The model under review builds one solid part; all positions refer to its coordinate system, in mm. A direction names the side the tool comes from. Round coordinates to 2 decimals unless told otherwise and drop trailing zeros. Loops run counter-clockwise (first coordinate to the right, second up) from the corner with the lowest first, then second, coordinate; pieces in that order, holes last. Notation, with made-up numbers: M 57.25,-31.5 L 70.25,-31.5 A25 cw 70.25,7.5 Z; hole C 48,-9 d6. An arc over 180 degrees is marked long. Return JSON: item names as keys, results as strings. Group by question number.
Q1. Draft analysis for pull direction Y (two halves, no side actions). For faces 1 (the face through (8.909, -0.885, 38.809)), 2 (the face through (-0.9, 8.91, 32.47)), 3 (the face through (7.9, -2.49, 11.74)), state which applies: pulls with the +Y half, pulls with the -Y half, needs draft (parallel to the pull), parting line crosses it, or undercut.
Q2. Consider section C-C (z = 13). State the section outline as (x, y) points.
Q3. Clearance check with flat-ended pins moving along their axes: pin 1 Ø4 at (x, y) = (5.5, 5) entering from +Z; pin 2 Ø2 at (y, z) = (-8, 47.5) entering from +X; pin 3 Ø1 at (x, y) = (0, -14) entering from -Z. State where each tip first meets the part, or that it passes through.
Q4. To check wall thickness, follow line 1 along Y through (x, z) = (5.25, 60.5); line 2 along Y through (x, z) = (0, 20); line 3 along Y through (x, z) = (-5.5, 10). State the ranges of each line that lie inside material, in increasing order.
Q5. For faces 4 (the face through (8, 41, 30.172)), 5 (the face through (6, 7, 49.212)), 6 (the face through (0, -8.282, 27)), 7 (the face through (4.3, -4.9, 61.912)), list the 3-axis set-ups (+Z, -Z, +X, -X, +Y, -Y) from which the entire face can be reached by the end or side of a thin tool; tool diameter is ignored.
Q6. Consider section B-B (y = 55). State the section outline as (x, z) points, and give its area (3 significant figures).
Autodesk Inventor part; units mm, degrees
ref_plane "YZ Plane" through (0, 0, 0) normal (1, 0, 0) x (0, 1, 0)
ref_plane "XZ Plane" through (0, 0, 0) normal (0, 1, 0) x (-1, 0, 0)
ref_plane "XY Plane" through (0, 0, 0) normal (0, 0, 1) x (1, 0, 0)
sketch "Sketch1" plane through (0, 0, 0) normal (0, 0, 1) x (1, 0, 0)
  circle A0 centre (0, 0) radius 6.35
  circle A1 centre (0, 0) radius 8.2824
  dimension "d0" = 12.7
extrude "Extrusion1" add sketch "Sketch1" along normal blind 23.8125
sketch "Sketch2" plane through (0, 0, 23.8125) normal (0, 0, 1) x (1, 0, 0)
  circle A0 centre (0, 0) radius 6.35
  circle A1 centre (0, 0) radius 8.2824
  line L0 (8.2824, 8.2824) -> (-8.2824, 8.2824)
  line L1 (-8.2824, -8.2824) -> (8.2824, -8.2824)
  line L2 (8.2824, -8.2824) -> (8.2824, 8.2824)
  line L3 (-8.2824, 8.2824) -> (-8.2824, -8.2824)
  circle A2 centre (0, 0) radius 6.35
extrude "Extrusion2" add sketch "Sketch2" along normal blind 25.4
sketch "Sketch3" plane through (0, 0, 49.2125) normal (0, 0, 1) x (1, 0, 0)
  circle A0 centre (0, 0) radius 6.35
  circle A1 centre (0, 0) radius 6.35
  circle A2 centre (0, 0) radius 8.2824
extrude "Extrusion3" add sketch "Sketch3" along normal blind 12.7
sketch "Sketch4" plane through (8.2824, -8.2824, 23.8125) normal (1, 0, 0) x (0, 0, -1)
  line L0 (-15.8821, 8.2824) -> (-14.086, 10.0784)
  line L1 (-15.8821, 8.2824) -> (-13.3421, 8.2824) construction
  line L2 (-14.086, 10.0784) -> (-14.086, 9.1804)
  line L3 (-15.8821, 8.2824) -> (-14.086, 6.4863)
  line L4 (-14.086, 6.4863) -> (-14.086, 7.3843)
  line L5 (-14.086, 7.3843) -> (-9.4174, 7.3843)
  line L6 (-9.4174, 7.3843) -> (-9.4174, 9.1804)
  line L7 (-9.4174, 9.1804) -> (-14.086, 9.1804)
  point P0 (23.8125, 8.2824)
  dimension "d7" = 2.54
  dimension "d8" = 45
extrude "Extrusion4" add sketch "Sketch4" along normal blind 1.27
sketch "Sketch5" plane through (0, 8.2824, 23.8125) normal (0, 1, 0) x (1, 0, 0)
  circle A0 centre (0, -12.7) radius 4.1412
  point P0 (0, 23.8125)
extrude "Extrusion5" add sketch "Sketch5" along normal blind 1.27
sketch "Sketch6" plane through (0, 9.5524, 36.5125) normal (0, 1, 0) x (1, 0, 0)
  circle A0 centre (0, 0) radius 4.1412
  circle A1 centre (0, 0) radius 7.62
  point P0 (0, 36.5125)
  dimension "d13" = 15.24
extrude "Extrusion6" add sketch "Sketch6" along normal blind 50.8 contours A0 | A1
sketch "Sketch7" plane through (0, 8.2824, 23.8125) normal (0, 1, 0) x (1, 0, 0)
  line L0 (8.2824, 0) -> (8.2824, -25.4)
  line L1 (8.2824, -19.0619) -> (8.2824, -6.3591)
  line L2 (8.2824, -6.3591) -> (7.0124, -6.3591)
  line L3 (7.0124, -6.3591) -> (7.0124, -19.0619)
  line L4 (7.0124, -19.0619) -> (8.2824, -19.0619)
  point P0 (0, 23.8125)
  dimension "d16" = 1.27
extrude "Extrusion7" add sketch "Sketch7" along normal blind 53.34
sketch "Sketch8" plane through (7.0124, 8.2824, 30.1716) normal (-1, 0, 0) x (0, 0, 1)
  line L0 (12.7028, 0) -> (12.7028, 53.34)
  line L1 (0, 53.34) -> (12.7028, 53.34)
  line L2 (12.7028, 53.34) -> (12.7028, 52.07)
  line L3 (12.7028, 52.07) -> (0, 52.07)
  line L4 (0, 52.07) -> (0, 53.34)
  point P0 (-30.1716, -8.2824)
  dimension "d19" = 1.27
extrude "Extrusion8" add sketch "Sketch8" along normal blind 12.7
sketch "Sketch9" plane through (-8.2824, -8.2824, 23.8125) normal (0, -1, 0) x (1, 0, 0)
  line L0 (0, 0) -> (0, 25.4)
  line L1 (16.5647, 0) -> (16.5647, 25.4)
  circle A0 centre (8.2824, 12.7) radius 8.2824
  line L2 (0, 21.8506) -> (16.5647, 21.8506)
  point P0 (8.2824, -23.8125)
revolve "Revolution1" add sketch "Sketch9" angle 45 about axis through (-8.2824, -8.2824, 45.6631) along (-1, 0, 0) contours A0
sketch "Sketch10" plane through (0, -14.7528, 39.1926) normal (0, -0.7071, 0.7071) x (-1, 0, 0)
  circle A0 centre (0, 0) radius 8.2824
  circle A1 centre (0, 0) radius 8.2824
  point P0 (0, 17.2816)
extrude "Extrusion9" add sketch "Sketch10" along normal blind 25.4
thread "Thread1"
properties part number "solenoid valve"
Values:
{
 "1": {"face 1": "pulls with the -Y half", "face 2": "undercut", "face 3": "parting line crosses it"},
 "2": {"outline": "C 0,0 d16.56; hole C 0,0 d12.7"},
 "3": {"pin 1": "stops at z = 61.91", "pin 2": "stops at x = 8.28", "pin 3": "stops at z = 29.03"},
 "4": {"line 1": "y = -29.37 to -27, -6.41 to -3.57, 3.57 to 6.41", "line 2": "y = -8.28 to -6.35, 6.35 to 8.28", "line 3": "y = -6.19 to -3.17, 3.17 to 6.19"},
 "5": {"face 4": "-Z, +X, +Y", "face 5": "+Z, +X, +Y", "face 6": "-Z, -Y", "face 7": "+Z, +X, -X, +Y"},
 "6": {"outline": "M 7.01,30.17 L 8.28,30.17 L 8.28,42.87 L 7.01,42.87 L 7.01,39.49 A7.62 ccw long 7.01,33.53 Z", "area": "196 mm2"}
}
